Geometry: final body of the model. Coordinates: model frame, mm. Face numbers are marked on the shaded views. A direction names the side the tool comes from. Coordinates: 2 decimals unless noted, no trailing zeros. Loops run counter-clockwise (first coordinate to the right, second up) from the corner with the lowest first, then second, coordinate; pieces in that order, holes last. Notation, with made-up numbers: (8.5, -28) - (17.5, -28) arc R34 cw to (17.5, 3) - close; hole circle Ø6 at (52, 38). An arc over 180 degrees is marked (long way). Answer in a Markdown table with one row per item.
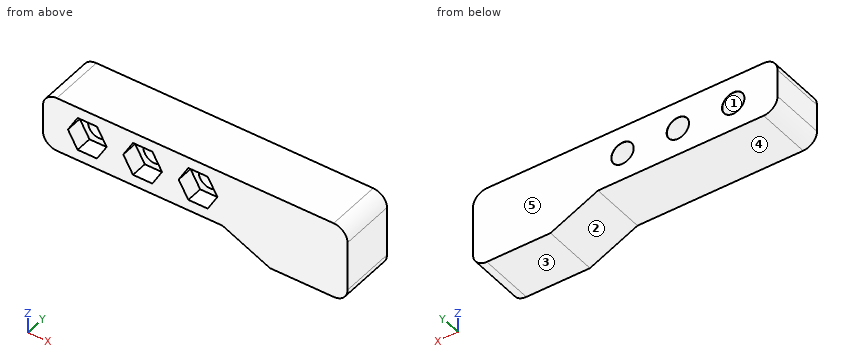
from build123d import *

# Parameters (mm, degrees)
BOSS_EXTRUDE1_DEPTH             = 10
F_4_0MM_DOWEL_HOLE1_D           = 4
F_4_0MM_DOWEL_HOLE1_CSINK_D     = 4.05
F_4_0MM_DOWEL_HOLE1_CSINK_ANGLE = 90
CUT_EXTRUDE1_DEPTH              = 3
FILLET1_R                       = 2.5


with BuildPart() as part:
    # Sketch1 → Boss-Extrude1 (new body)
    with BuildSketch(Plane(origin=(0, 0, 0), x_dir=(1, 0, 0), z_dir=(0, 1, 0))):
        Polygon((0, 5), (0, -5), (55, -5), (55, 9), (41, 9), (32.421972318, 5), align=None)
    extrude(amount=BOSS_EXTRUDE1_DEPTH)

    # Ø4.0mm Dowel Hole1 (through all)
    with Locations(Plane(origin=(0, 10, 0), x_dir=(1, 0, 0), z_dir=(0, 1, 0))):
        with Locations((8, 0), (18, 0), (28, 0)):
            CounterSinkHole(F_4_0MM_DOWEL_HOLE1_D / 2, F_4_0MM_DOWEL_HOLE1_CSINK_D / 2, counter_sink_angle=F_4_0MM_DOWEL_HOLE1_CSINK_ANGLE)

    # Sketch5 → Cut-Extrude1 (cut)
    with BuildSketch(Plane.XZ):
        Polygon((9.75, -3.031088913), (11.5, 0), (9.75, 3.031088913), (6.25, 3.031088913), (4.5, 0), (6.25, -3.031088913), align=None)
        Polygon((21.5, 0), (19.75, 3.031088913), (16.25, 3.031088913), (14.5, 0), (16.25, -3.031088913), (19.75, -3.031088913), align=None)
        Polygon((31.5, 0), (29.75, 3.031088913), (26.25, 3.031088913), (24.5, 0), (26.25, -3.031088913), (29.75, -3.031088913), align=None)
    extrude(amount=-CUT_EXTRUDE1_DEPTH, mode=Mode.SUBTRACT)

    # Fillet1
    fillet1_edges = [part.edges().sort_by_distance(p)[0] for p in [
        (55, 5, -9),
        (55, 5, 5),
        (0, 5, 5),
        (0, 5, -5),
    ]]
    fillet(fillet1_edges, radius=FILLET1_R)


solid = part.part
(1) Access query for the marked faces 4 and 5. Directions: +Z, -Z, +X, -X, +Y, -Y. A direction counts if a zero-diameter tool reaches every point of the face in a straight line with its end or side. Return the directions, or none.
Verdict:
| item | result |
|---|---|
| face 4 | -Z, -X, +Y, -Y |
| face 5 | +Z, -Z, +X, -X, +Y |
(2) Cut plane C-C on y = 9.25. Output: boundary loops of the cut face in (x, z).
Verdict:
| item | result |
|---|---|
| outline | (0, -2.5) arc R2.5 ccw to (2.5, -5) - (32.42, -5) - (41, -9) - (52.5, -9) arc R2.5 ccw to (55, -6.5) - (55, 2.5) arc R2.5 ccw to (52.5, 5) - (2.5, 5) arc R2.5 ccw to (0, 2.5) - close; hole circle Ø4 at (8, 0); hole circle Ø4 at (18, 0); hole circle Ø4 at (28, 0) |
(3) Pull-direction query (X, two-part tool) for the marked faces 1, 2 and 3; classes: pulls with the +X half, pulls with the -X half, needs draft (parallel to the pull), parting line crosses it, or undercut.
Verdict:
| item | result |
|---|---|
| face 1 | undercut |
| face 2 | pulls with the -X half |
| face 3 | needs draft |
(4) Cut plane A-A on x = 8. Output: boundary loops of the cut face in (y, z) (3 decimals).
Verdict:
| item | result |
|---|---|
| outline | (0, -5) - (10, -5) - (10, -2.025) - (9.975, -2) - (3, -2) - (3, -3.031) - (0, -3.031) - close; (0, 3.031) - (3, 3.031) - (3, 2) - (9.975, 2) - (10, 2.025) - (10, 5) - (0, 5) - close |
(5) Cut plane B-B on y = 2.5. Output: boundary loops of the cut face in (x, z).
Verdict:
| item | result |
|---|---|
| outline | (0, -2.5) arc R2.5 ccw to (2.5, -5) - (32.42, -5) - (41, -9) - (52.5, -9) arc R2.5 ccw to (55, -6.5) - (55, 2.5) arc R2.5 ccw to (52.5, 5) - (2.5, 5) arc R2.5 ccw to (0, 2.5) - close; hole (4.5, 0) - (6.25, -3.03) - (9.75, -3.03) - (11.5, 0) - (9.75, 3.03) - (6.25, 3.03) - close; hole (14.5, 0) - (16.25, -3.03) - (19.75, -3.03) - (21.5, 0) - (19.75, 3.03) - (16.25, 3.03) - close; hole (24.5, 0) - (26.25, -3.03) - (29.75, -3.03) - (31.5, 0) - (29.75, 3.03) - (26.25, 3.03) - close |
(6) First-contact query: pin 1 Ø1.8 at (x, z) = (28.5, -1.5) entering from -Y; pin 2 Ø1 at (x, y) = (39, 6.5) entering from -Z; pin 3 Ø2.5 at (x, y) = (18.5, 1) entering from -Z. Flat tips, straight axial feed; report the tip coordinate or a pass-through.
Verdict:
| item | result |
|---|---|
| pin 1 | stops at y = 3 |
| pin 2 | stops at z = -8.3 |
| pin 3 | stops at z = -5 |
(7) Ray query, probe 1 along Z at (x, y) = (28, 7); probe 2 along Y at (x, z) = (20, 1.25); probe 3 along Z at (x, y) = (14, 5.5). Return the intervals inside material, ascending.
Verdict:
| item | result |
|---|---|
| probe 1 | z = -5 to -2, 2 to 5 |
| probe 2 | y = 3 to 10 |
| probe 3 | z = -5 to 5 |
(8) Cut plane D-D on z = -0.5. State how many separate pieces and enclosed holes the cut face has, then the cut area to 3 significant figures.
Verdict:
| item | result |
|---|---|
| separate pieces | 4 |
| enclosed holes | 0 |
| area | 411 mm² |
